Could you check a few things on this model? Use its own coordinates, in mm. Give positions to 0.01 mm unless a question says otherwise; leave off trailing zeros. Order: outer loops, then holes, each group sorted by start corner. A loop starts at its lowest first (then second) coordinate and runs counter-clockwise, first axis right, second up.
(1) Will this pin go through, and if not, where does the flat tip stop? pin 1 (2.5 mm diameter, centred on y = -65, z = 5, fed in from -X).
(2) Imagine slicing it at B-B, the plane x = 35.55. Write out the boundary of the cut face in (y, z).
(3) Imagine slicing it at A-A, the plane z = 15. Write out the boundary of the cut face in (x, y).
(4) Imagine slicing it at D-D, the plane z = 5. Write out the boundary of the cut face in (x, y), then the cut area to 3 significant figures.
(5) If we mould it in two halves opening along Z, with no side actions, what happens to faces 1 (the cylindrical face through (34.52, -67.95, 14.54)), 2 (the flat face through (35, -80, -18)), 3 (the flat face through (35, -70, 20))? For each: released by +Z, released by -Z, zero draft, split by the parting line, or undercut.
(6) Imagine slicing it at C-C, the plane y = -65. Write out the boundary of the cut face in (x, z), then the cut area to 3 significant figures.
(7) If I drill on probe 1 along Z at (x, y) = (34.8, -70); probe 2 along Y at (x, z) = (33.75, 5); probe 3 along Z at (x, y) = (33.4, -71.75), over which ranges is the centre line in solid material (lowest first)?
from build123d import *

# Parameters (mm, degrees)
SKETCH_1_W      = 78
SKETCH_1_H      = 20
SKETCH_1_R      = 2.1
EXTRUDE_1_DEPTH = 3


with BuildPart() as part:
    # 草图1 → 凸台-拉伸1 (new body)
    with BuildSketch(Plane(origin=(36, 0, 0), x_dir=(0, 0, -1), z_dir=(1, 0, 0))):
        with Locations((19, -70)):
            Rectangle(SKETCH_1_W, SKETCH_1_H)
        with Locations(Location((-15, -70, 0), (0, 0, 180))):
            Circle(SKETCH_1_R, mode=Mode.SUBTRACT)
        with Locations(Location((41, -70, 0), (0, 0, 180))):
            Circle(SKETCH_1_R, mode=Mode.SUBTRACT)
        with Locations(Location((51, -70, 0), (0, 0, 180))):
            Circle(SKETCH_1_R, mode=Mode.SUBTRACT)
        with Locations(Location((26, -70, 0), (0, 0, 180))):
            Circle(SKETCH_1_R, mode=Mode.SUBTRACT)
        with Locations(Location((16, -70, 0), (0, 0, 180))):
            Circle(SKETCH_1_R, mode=Mode.SUBTRACT)
        with Locations(Location((-5, -65, 0), (0, 0, 180))):
            Circle(SKETCH_1_R, mode=Mode.SUBTRACT)
        with Locations(Location((-5, -75, 0), (0, 0, 180))):
            Circle(SKETCH_1_R, mode=Mode.SUBTRACT)
    extrude(amount=-EXTRUDE_1_DEPTH)


solid = part.part
Answer block:
1. pin 1: passes through
2. outline: (-80, -58) - (-60, -58) - (-60, 20) - (-80, 20) - close; hole circle Ø4.2 at (-75, 5); hole circle Ø4.2 at (-70, -51); hole circle Ø4.2 at (-70, -41); hole circle Ø4.2 at (-70, -26); hole circle Ø4.2 at (-70, -16); hole circle Ø4.2 at (-70, 15); hole circle Ø4.2 at (-65, 5)
3. outline: (33, -80) - (36, -80) - (36, -72.1) - (33, -72.1) - close; (33, -67.9) - (36, -67.9) - (36, -60) - (33, -60) - close
4. outline: (33, -80) - (36, -80) - (36, -77.1) - (33, -77.1) - close; (33, -72.9) - (36, -72.9) - (36, -67.1) - (33, -67.1) - close; (33, -62.9) - (36, -62.9) - (36, -60) - (33, -60) - close
4. area: 34.8 mm2
5. face 1: undercut
5. face 2: zero draft
5. face 3: released by +Z
6. outline: (33, -58) - (36, -58) - (36, 2.9) - (33, 2.9) - close; (33, 7.1) - (36, 7.1) - (36, 20) - (33, 20) - close
6. area: 221 mm2
7. probe 1: z = -58 to -53.1, -48.9 to -43.1, -38.9 to -28.1, -23.9 to -18.1, -13.9 to 12.9, 17.1 to 20
7. probe 2: y = -80 to -77.1, -72.9 to -67.1, -62.9 to -60
7. probe 3: z = -58 to -52.16, -49.84 to -42.16, -39.84 to -27.16, -24.84 to -17.16, -14.84 to 13.84, 16.16 to 20
